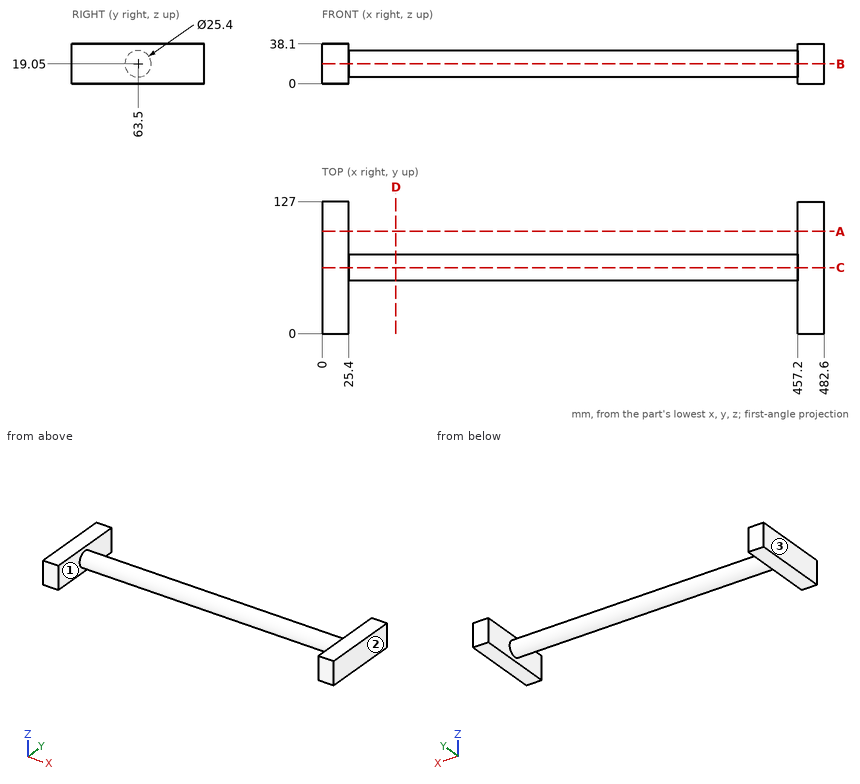
Input: dimensioned drawing with shaded views. Units: mm. Origin: part minimum x, y, z. Give positions to 0.01 mm unless a question says otherwise; leave off trailing zeros. Write each loop counter-clockwise with the first axis right and the second up, starting at its lowest first coordinate (ties: lowest second). Pieces come first, ordered by that corner, then holes. Notation, with made-up numbers: (61, -32.75) - (100, -32.75) arc R12 ccw to (100, -23.75) - close; hole circle Ø10 at (-25.75, 6.25). An arc over 180 degrees is marked (long way). One line per item, written item: value. Start each with the question number.
Q1. Section query B-B, the plane z = 19.05. Return the cut outline in (x, y).
Q2. Section query A-A, the plane y = 98.5. Return the cut outline in (x, z), then the cut area to 3 significant figures.
Q3. Section query C-C, the plane y = 63.5. Return the cut outline in (x, z).
Q4. First-contact query: pin 1 Ø3 at (x, z) = (234, 30.5) entering from -Y; pin 2 Ø8 at (x, z) = (75.5, 9.5) entering from +Y; pin 3 Ø1.5 at (x, z) = (127, 20.5) entering from +Y. Flat tips, straight axial feed; report the tip coordinate or a pass-through.
Q5. Material intervals for probe 1 along X at (y, z) = (19.5, 31.5); probe 2 along Y at (x, z) = (346, 19.5); probe 3 along Y at (x, z) = (288, 29), sorted ascending. Write a range as from..to.
Q6. Draft query along X for the marked faces 1, 2 and 3. Return one class per face: +X half, -X half, draft (parallel to the pull), parting line (faces both ways), or undercut.
Q7. Section query D-D, the plane x = 71. Return the cut outline in (y, z).
Answer:
1. outline: (0, 0) - (25.4, 0) - (25.4, 50.8) - (457.2, 50.8) - (457.2, 0) - (482.6, 0) - (482.6, 127) - (457.2, 127) - (457.2, 76.2) - (25.4, 76.2) - (25.4, 127) - (0, 127) - close
2. outline: (0, 0) - (25.4, 0) - (25.4, 38.1) - (0, 38.1) - close; (457.2, 0) - (482.6, 0) - (482.6, 38.1) - (457.2, 38.1) - close
2. area: 1,940 mm2
3. outline: (0, 0) - (25.4, 0) - (25.4, 6.35) - (457.2, 6.35) - (457.2, 0) - (482.6, 0) - (482.6, 38.1) - (457.2, 38.1) - (457.2, 31.75) - (25.4, 31.75) - (25.4, 38.1) - (0, 38.1) - close
4. pin 1: stops at y = 55.61
4. pin 2: stops at y = 74.92
4. pin 3: stops at y = 76.18
5. probe 1: x = 0..25.4, 457.2..482.6
5. probe 2: y = 50.81..76.19
5. probe 3: y = 55.61..71.39
6. face 1: undercut
6. face 2: +X half
6. face 3: -X half
7. outline: circle Ø25.4 at (63.5, 19.05)
